For this review, use the dimensioned drawing (mm, ordinates from the lowest corner) and the shaded views. Coordinates: 2 decimals unless noted, no trailing zeros. Loops run counter-clockwise (first coordinate to the right, second up) from the corner with the lowest first, then second, coordinate; pieces in that order, holes last. Notation, with made-up numbers: (-22, 87) -> (-1, 87) arc R9 ccw to (-1, 99) -> close; hole circle Ø5 at (1.5, -32). An arc over 180 degrees is marked (long way). Answer as a JSON object with one key per item and string values.
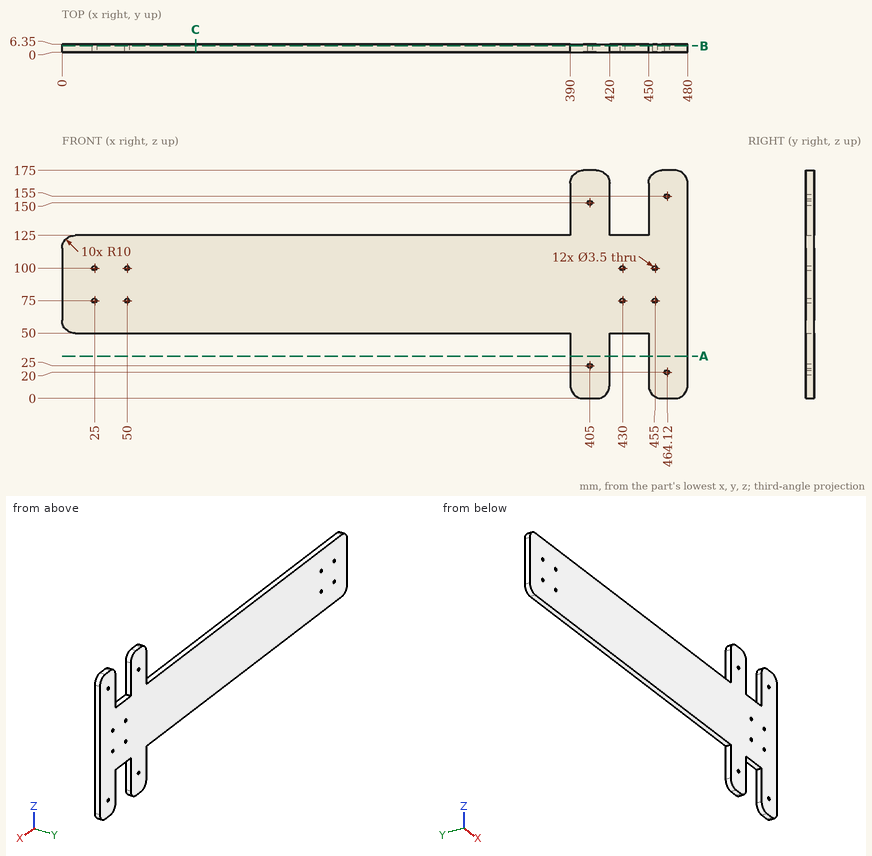
1) Add section A-A, the plane z = 32.5. Give the boundary of the cut face in (x, y).
Completed:
{"outline": "(390, 0) -> (420, 0) -> (420, 6.35) -> (390, 6.35) -> close; (450, 0) -> (480, 0) -> (480, 6.35) -> (450, 6.35) -> close"}
2) Clearance check with flat-ended pins moving along their axes: pin 1 Ø1.5 at (x, y) = (388, 4.5) entering from +Z; pin 2 Ø3 at (y, z) = (3, 154.5) entering from -X. State where each tip first meets the part, or that it passes through.
Completed:
{"pin 1": "z = 125", "pin 2": "x = 390"}
3) Wall thickness on probe 1 along X at (y, z) = (4.5, 75); probe 2 along Z at (x, y) = (25, 1.5); probe 3 along X at (y, z) = (1, 143.5): over which ranges is each line inside the solid? List them lowest first.
Completed:
{"probe 1": "0 to 23.25, 26.75 to 48.25, 51.75 to 428.25, 431.75 to 453.25, 456.75 to 480", "probe 2": "50 to 73.25, 76.75 to 98.25, 101.75 to 125", "probe 3": "390 to 420, 450 to 480"}
4) Add section B-B, the plane y = 5. Count the separate pieces of the cut face and the enclosed holes in it, and give its area (3 significant figures).
Completed:
{"separate pieces": "1", "enclosed holes": "12", "area": "41,700 mm²"}
5) Add section C-C, the plane x = 102.5. Give the boundary of the cut face in (y, z).
Completed:
{"outline": "(0, 50) -> (6.35, 50) -> (6.35, 125) -> (0, 125) -> close"}
